```python
from build123d import *

# Parameters (mm, degrees)
F0_R      = 9.25
F1_DEPTH  = 3
F1_FACE_R = 9.25
F2_DEPTH  = 3
F2_TAPER  = 15
F2_FACE_R = 8.4461524227
F3_DEPTH  = 15
F3_TAPER  = 2


with BuildPart() as f1:
    # F0 (on Top) → F1 (new body)
    with BuildSketch(Plane.XY):
        Circle(F0_R)
    extrude(amount=F1_DEPTH)

    # F1_face (on face) → F2 (join)
    with BuildSketch(Plane.XY.offset(3)):
        Circle(F1_FACE_R)
    extrude(amount=F2_DEPTH, taper=F2_TAPER)

    # F2_face (on face) → F3 (join)
    with BuildSketch(Plane.XY.offset(6)):
        Circle(F2_FACE_R)
    extrude(amount=F3_DEPTH, taper=F3_TAPER)


solid = f1.part
```
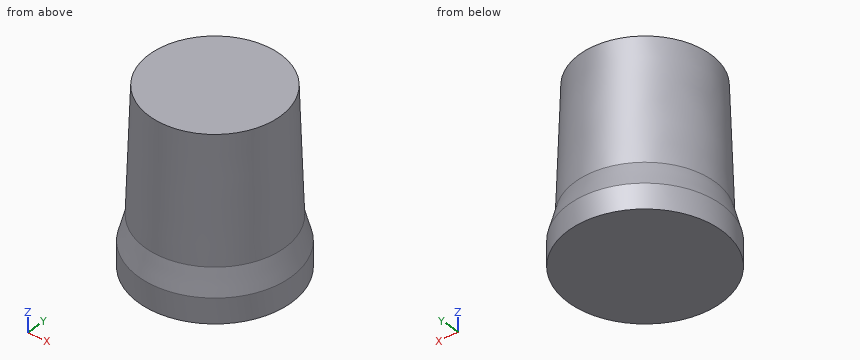
Check sheet for the modelled part. Datum: model origin and axes. Units: mm. Round coordinates to 2 decimals unless told otherwise and drop trailing zeros. Order: outer loops, then holes, each group sorted by start corner. A loop starts at its lowest first (then second) coordinate and runs counter-clockwise, first axis right, second up. Notation, with made-up numbers: (-27.75, -10) - (-19.75, -10) arc R31 cw to (-19.75, 15) - close; hole circle Ø10 at (43.25, 44). An arc over 180 degrees is marked (long way). Write item = value, one per line.
Q1. Section check D-D (z = 17). Record the boundary of the cut face in (x, y), and give its area (3 significant figures).
Computed:
outline = circle Ø16.12 at (0, 0)
area = 204 mm^2
Q2. Thickness scan on line 1 along X through (y, z) = (-1, 6.25); line 2 along Y through (x, z) = (-7.75, 3); line 3 along X through (y, z) = (-6.25, 10). Record the ranges inside material, lowest first.
Computed:
line_1 = -8.38 to 8.38
line_2 = -5.05 to 5.05
line_3 = -5.47 to 5.47
Q3. Section check C-C (z = 11.25). Record the boundary of the cut face in (x, y).
Computed:
outline = circle Ø16.53 at (0, 0)
Q4. Section check A-A (y = 0). Record the boundary of the cut face in (x, z), and give its area (3 significant figures).
Computed:
outline = (-9.25, 0) - (9.25, 0) - (9.25, 3) - (8.45, 6) - (7.92, 21) - (-7.92, 21) - (-8.45, 6) - (-9.25, 3) - close
area = 354 mm^2
Q5. Go/stop test with flat-tipped pins: pin 1 (6 mm diameter, centred on y = 6.5, z = 7.5, fed in from -X); pin 2 (6 mm diameter, centred on x = -4.5, z = 7, fed in from -Y); pin 3 (10 mm diameter, centred on y = -0.5, z = 12, fed in from -X). Record where each tip stops, or that it passes through.
Computed:
pin_1 = -7.63
pin_2 = -8.42
pin_3 = -8.41
